Part print with two shaded views. Sizes in mm from the minimum x, y, z corner. Round coordinates to 2 decimals unless told otherwise and drop trailing zeros. Order: outer loops, then holes, each group sorted by start corner. A loop starts at its lowest first (then second) coordinate and runs counter-clockwise, first axis right, second up. Notation, with made-up numbers: M 19.25,16 L 78.25,16 A18 ccw 78.25,26 Z; hole C 35.5,-7.5 d4. An arc over 180 degrees is marked long. Return JSON: item names as keys, results as strings. Group by question number.
Item 1: Slice it at A-A on y = 0.3. Give the number of separate pieces and of enclosed holes in the cut face, then the cut area to 3 significant figures.
Item 2: Slice it at C-C on z = 46.5. Write the cut outline in (x, y).
Item 3: Slice it at B-B on x = 49. Write the cut outline in (y, z).
Item 4: Probe line 1 along X through (y, z) = (0.1, 52.5) (1 decimal); line 2 along Z through (x, y) = (51, 0.4) (1 decimal); line 3 along X through (y, z) = (0.1, 53) (1 decimal). List the from-to ranges inside material, lowest first.
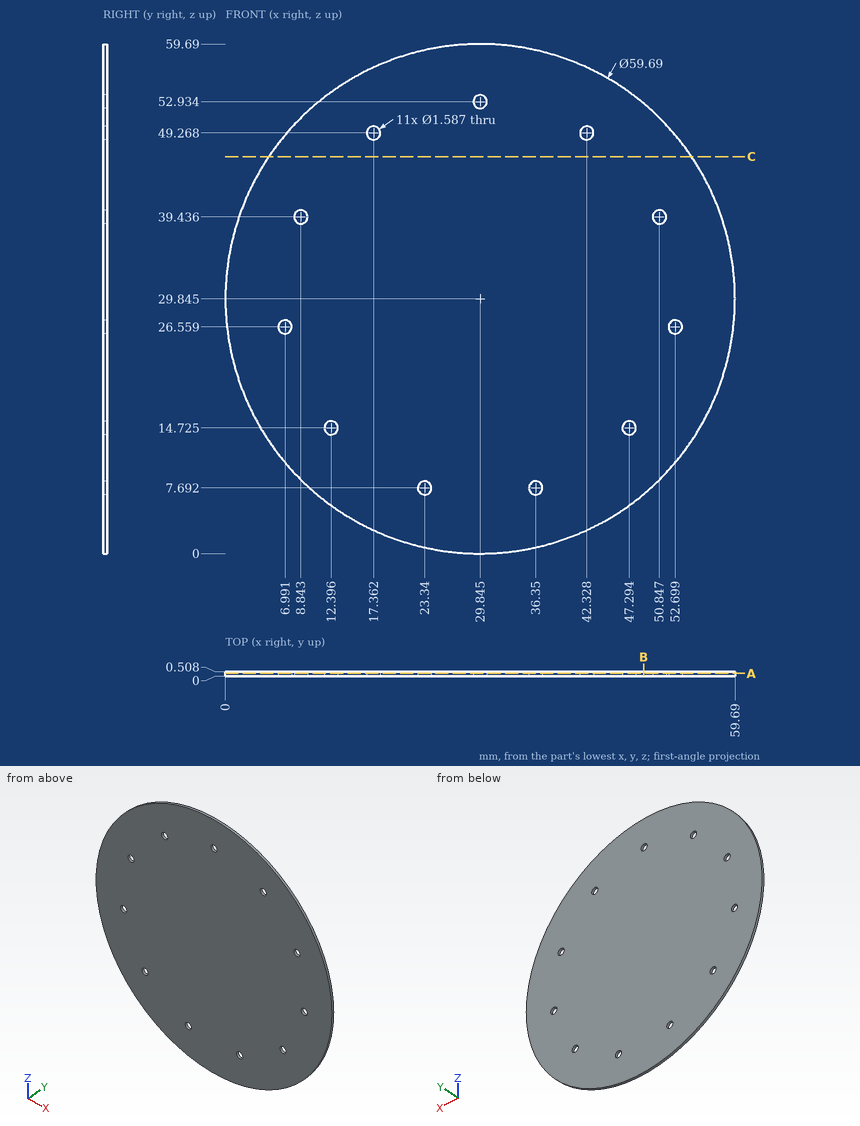
Output values:
{
 "1": {"separate pieces": "1", "enclosed holes": "11", "area": "2,780 mm²"},
 "2": {"outline": "M 5.08,0 L 54.61,0 L 54.61,0.51 L 5.08,0.51 Z"},
 "3": {"outline": "M 0,6.96 L 0.51,6.96 L 0.51,52.73 L 0,52.73 Z"},
 "4": {"line 1": "10.4 to 29.2, 30.5 to 49.3", "line 2": "8.8 to 38.7, 40.2 to 50.9", "line 3": "11 to 29.1, 30.6 to 48.7"}
}
